from build123d import *

# Parameters (mm, degrees)
SKETCH1_R           = 9.525
BOSS_EXTRUDE1_DEPTH = 67.46875
SKETCH2_R           = 9.525
SKETCH2_R_2         = 9.025
CUT_EXTRUDE1_DEPTH  = 57.15


with BuildPart() as part:
    # Sketch1 → Boss-Extrude1 (new, symmetric)
    with BuildSketch(Plane(origin=(0, 0, 0), x_dir=(0, 0, -1), z_dir=(1, 0, 0))):
        Circle(SKETCH1_R)
    extrude(amount=BOSS_EXTRUDE1_DEPTH, both=True)

    # Sketch2 → Cut-Extrude1 (cut, symmetric)
    with BuildSketch(Plane(origin=(0, 0, 0), x_dir=(0, 0, -1), z_dir=(1, 0, 0))):
        Circle(SKETCH2_R)
        Circle(SKETCH2_R_2, mode=Mode.SUBTRACT)
    extrude(amount=CUT_EXTRUDE1_DEPTH, both=True, mode=Mode.SUBTRACT)


solid = part.part
Model file for the job. Use its own axes, mm. A direction names the side the tool comes from. Coordinates: 2 decimals unless noted, no trailing zeros. Write each loop counter-clockwise with the first axis right and the second up, starting at its lowest first coordinate (ties: lowest second). Pieces come first, ordered by that corner, then holes. Notation, with made-up numbers: (-26.75, 42) -> (-5.75, 42) arc R18 cw to (-5.75, 54) -> close; hole circle Ø8 at (-36, 2). An arc over 180 degrees is marked (long way). One line per item, written item: value. Start each with the question number.
1) Probe probe 1 along X at (y, z) = (7.25, 5.75); probe 2 along Y at (x, z) = (-17, 0.25); probe 3 along Y at (x, z) = (-62, 4.5). List the from-to ranges inside material, lowest first.
2) Slice it at C-C on x = 5.5. Write the cut outline in (y, z) (3 decimals).
3) Which spindle directions (+Z, -Z, +X, -X, +Y, -Y) get a long thin tool onto all of the face, cutting with end or side? Do faces 1 (the face through (-62.237, -5.796, 7.559)), 2 (the face through (-0.8, -8.8, 2)). Say none if no direction does.
4) Pull direction X, two halves, no side cores. Call faces 3 (the face through (57.15, 6, -7)), 4 (the face through (-57.15, 6, -7)), 5 (the face through (62.382, -5.796, 7.559)), 6 (the face through (-67.469, 0, 0)): +X half, -X half, draft (parallel to the pull), parting line (faces both ways), or undercut.
5) Slice it at A-A on z = 0. Write the cut outline in (x, y) (3 decimals), then the cut area to 3 significant figures.
6) Flat gauge pins, fed straight in: pin 1 Ø5 at (x, z) = (5.5, 1) entering from -Y (3 decimals); pin 2 Ø1 at (x, y) = (48.5, 1) entering from +Z; pin 3 Ø3 at (x, y) = (-17, 1) entering from -Z (3 decimals). Where does each tip first touch, or does it go through?
Answers follow:
1. probe 1: -67.47 to -57.15, 57.15 to 67.47
1. probe 2: -9.02 to 9.02
1. probe 3: -8.39 to 8.39
2. outline: circle Ø18.05 at (0, 0)
3. face 1: +X, -X
3. face 2: none
4. face 3: undercut
4. face 4: undercut
4. face 5: draft
4. face 6: -X half
5. outline: (-67.469, -9.525) -> (-57.15, -9.525) -> (-57.15, -9.025) -> (57.15, -9.025) -> (57.15, -9.525) -> (67.469, -9.525) -> (67.469, 9.525) -> (57.15, 9.525) -> (57.15, 9.025) -> (-57.15, 9.025) -> (-57.15, 9.525) -> (-67.469, 9.525) -> close
5. area: 2,460 mm2
6. pin 1: y = -9.025
6. pin 2: z = 9.01
6. pin 3: z = -9.025
